```python
from build123d import *

# Parameters (mm, degrees)
SKETCH1_W           = 20
SKETCH1_H           = 11
BOSS_EXTRUDE1_DEPTH = 6
SHELL1_T            = -1
SKETCH2_R           = 1.9939
BOSS_EXTRUDE2_DEPTH = 6.35
SKETCH3_R           = 0.875
CUT_EXTRUDE1_DEPTH  = 24.963513933


with BuildPart() as part:
    # Sketch1 → Boss-Extrude1 (new, symmetric)
    with BuildSketch(Plane.XY):
        with Locations((10, 0)):
            Rectangle(SKETCH1_W, SKETCH1_H)
    extrude(amount=BOSS_EXTRUDE1_DEPTH, both=True)

    # Shell1
    shell1_openings = [part.faces().sort_by_distance(p)[0] for p in [
        (10, 5.5, 0),
        (10, -5.5, 0),
    ]]
    offset(amount=SHELL1_T, openings=shell1_openings, kind=Kind.INTERSECTION)

    # Sketch2 → Boss-Extrude2 (add)
    with BuildSketch(Plane.ZY):
        Circle(SKETCH2_R)
    extrude(amount=BOSS_EXTRUDE2_DEPTH)

    # Sketch3 → Cut-Extrude1 (cut, through all)
    with BuildSketch(Plane.XY.offset(6)):
        with Locations((5, 3)):
            Circle(SKETCH3_R)
        with Locations((15, -3)):
            Circle(SKETCH3_R)
    extrude(amount=-CUT_EXTRUDE1_DEPTH, mode=Mode.SUBTRACT)


solid = part.part
```
Could you check a few things on this model? Use its own coordinates, in mm. A direction names the side the tool comes from. Give positions to 0.01 mm unless a question says otherwise; leave off trailing zeros. Write each loop counter-clockwise with the first axis right and the second up, starting at its lowest first coordinate (ties: lowest second). Pieces come first, ordered by that corner, then holes. Notation, with made-up numbers: (85.5, 56) - (109.5, 56) arc R14 cw to (109.5, 66) - close; hole circle Ø7 at (-38, -5). An arc over 180 degrees is marked (long way). One line per item, written item: value. Start each with the question number.
Item 1: Imagine slicing it at D-D, the plane y = 0. List the corners of the cut face in (x, z) for me.
Item 2: Imagine slicing it at A-A, the plane z = 0. List the corners of the cut face in (x, y) for me, and give its area (3 significant figures).
Item 3: Which directions (+Z, -Z, +X, -X, +Y, -Y) give clear straight access to the entire face, cutting with the end or side of a thin tool? Please do faces 1 (the face through (19, 0, 0)), 2 (the face through (14.126, -2.962, -5.493)), 3 (the face through (-3.1, 0.6, 1.9)).
Item 4: Please list where these lines run through material, in increasing order: line 1 (Z direction, x = 14.5, y = -1.75); line 2 (Y direction, x = 5, z = 5.8) (3 decimals); line 3 (Y direction, x = 15, z = 5.25) (3 decimals). Write a range as from..to.
Item 5: I'm going to push a flat-ended pin straight in: pin 1 (4 mm diameter, centred on y = 3.5, z = 0.5, fed in from -X). Where does the tip first touch, or does it pass through?
Item 6: Imagine slicing it at B-B, the plane y = -3. List the corners of the cut face in (x, z) for me (3 decimals).
Item 7: Imagine slicing it at C-C, the plane x = 5. List the corners of the cut face in (y, z) for me (3 decimals).
Item 8: If we mould it in two halves opening along Y, with no side actions, what happens to faces 4 (the face through (9.2, 5.5, -5.3)), 5 (the face through (5.4, 2.22, -5.49)), 6 (the face through (10, 0, 5)), 7 (the face through (14.126, -2.962, 5.507))? For each: +Y half, -Y half, draft (parallel to the pull), parting line (faces both ways), or undercut.
Geometry says:
1. outline: (-6.35, -1.99) - (0, -1.99) - (0, -6) - (20, -6) - (20, 6) - (0, 6) - (0, 1.99) - (-6.35, 1.99) - close; hole (1, -5) - (19, -5) - (19, 5) - (1, 5) - close
2. outline: (-6.35, -1.99) - (0, -1.99) - (0, -5.5) - (1, -5.5) - (1, 5.5) - (0, 5.5) - (0, 1.99) - (-6.35, 1.99) - close; (19, -5.5) - (20, -5.5) - (20, 5.5) - (19, 5.5) - close
2. area: 47.3 mm^2
3. face 1: +Y, -Y
3. face 2: +Z, -Z
3. face 3: -X
4. line 1: -6..-5, 5..6
4. line 2: -5.5..2.125, 3.875..5.5
4. line 3: -5.5..-3.875, -2.125..5.5
5. pin 1: x = -6.35
6. outline: (0, -6) - (14.125, -6) - (14.125, -5) - (1, -5) - (1, 5) - (14.125, 5) - (14.125, 6) - (0, 6) - close; (15.875, -6) - (20, -6) - (20, 6) - (15.875, 6) - (15.875, 5) - (19, 5) - (19, -5) - (15.875, -5) - close
7. outline: (-5.5, -6) - (2.125, -6) - (2.125, -5) - (-5.5, -5) - close; (-5.5, 5) - (2.125, 5) - (2.125, 6) - (-5.5, 6) - close; (3.875, -6) - (5.5, -6) - (5.5, -5) - (3.875, -5) - close; (3.875, 5) - (5.5, 5) - (5.5, 6) - (3.875, 6) - close
8. face 4: +Y half
8. face 5: undercut
8. face 6: draft
8. face 7: undercut
